from build123d import *

# Parameters (mm, degrees)
SKETCH1_R           = 2.4765
BOSS_EXTRUDE1_DEPTH = 1.524
SKETCH2_R           = 1.524
BOSS_EXTRUDE2_DEPTH = 18.161
CUT_EXTRUDE1_START  = -1.397
SKETCH4_R           = 1.524
CUT_EXTRUDE1_DEPTH  = 1.397
SKETCH5_R           = 1.4605
BOSS_EXTRUDE3_DEPTH = 0.381
SKETCH6_R           = 1.524
BOSS_EXTRUDE4_DEPTH = 1.016
FILLET1_R           = 0.635


with BuildPart() as part:
    # Sketch1 → Boss-Extrude1 (new body)
    with BuildSketch(Plane.XY):
        Circle(SKETCH1_R)
    extrude(amount=-BOSS_EXTRUDE1_DEPTH)

    # Sketch2 → Boss-Extrude2 (add)
    with BuildSketch(Plane(origin=(0, 0, -1.524), x_dir=(-1, 0, 0), z_dir=(0, 0, -1))):
        with Locations(Location((0, 0, 0), (0, 0, 180))):
            Circle(SKETCH2_R)
    extrude(amount=BOSS_EXTRUDE2_DEPTH)

    # Sketch4 → Cut-Extrude1 (cut)
    with BuildSketch(Plane(origin=(0, 0, -19.685), x_dir=(-1, 0, 0), z_dir=(0, 0, -1)).offset(CUT_EXTRUDE1_START)):
        with Locations(Location((0, 0, 0), (0, 0, 180))):
            Circle(SKETCH4_R)
    extrude(amount=CUT_EXTRUDE1_DEPTH, mode=Mode.SUBTRACT)

    # Sketch5 → Boss-Extrude3 (add)
    with BuildSketch(Plane(origin=(0, 0, -18.288), x_dir=(-1, 0, 0), z_dir=(0, 0, -1))):
        with Locations(Location((0, 0, 0), (0, 0, 180))):
            Circle(SKETCH5_R)
    extrude(amount=BOSS_EXTRUDE3_DEPTH)

    # Sketch6 → Boss-Extrude4 (add)
    with BuildSketch(Plane(origin=(0, 0, -18.669), x_dir=(-1, 0, 0), z_dir=(0, 0, -1))):
        with Locations(Location((0, 0, 0), (0, 0, 180))):
            Circle(SKETCH6_R)
    extrude(amount=BOSS_EXTRUDE4_DEPTH)

    # Fillet1
    fillet1_edges = [part.edges().sort_by_distance(p)[0] for p in [
        (-2.4765, 0, 0),
        (-2.4765, 0, -1.524),
    ]]
    fillet(fillet1_edges, radius=FILLET1_R)


solid = part.part
Check sheet for the modelled part. Datum: model origin and axes. Units: mm. A direction names the side the tool comes from. Give positions to 0.01 mm unless a question says otherwise; leave off trailing zeros. Write each loop counter-clockwise with the first axis right and the second up, starting at its lowest first coordinate (ties: lowest second). Pieces come first, ordered by that corner, then holes. Notation, with made-up numbers: (79, 35) -> (135, 35) arc R14 cw to (135, 45) -> close; hole circle Ø6 at (60.25, 4.25). An arc over 180 degrees is marked (long way). Write item = value, one per line.
Item 1: Sectioned sample at C-C on z = -10.5. Record the boundary of the cut face in (x, y).
Output:
outline = circle Ø3.05 at (0, 0)
Item 2: Release check for a two-part mould opening along Z. For faces 1 (the flat face through (0, 0, -19.685)), 2 (the cylindrical face through (-1.16, 0.89, -18.48)), 3 (the cylindrical face through (-0.2, -1.51, -9.79)) record: +Z half, -Z half, draft (parallel to the pull), parting line (faces both ways), or undercut.
Output:
face_1 = -Z half
face_2 = undercut
face_3 = draft
Item 3: Gauge pin test, flat end, axial feed: pin 1 (1.5 mm diameter, centred on y = 1, z = -8.5, fed in from -X). Record the tip position at first contact, or that the pin passes through.
Output:
pin_1 = -1.5
Item 4: Tool access check on faces 4 (the flat face through (0, 0, 0)), 5 (the cylindrical face through (-0.2, -1.51, -19.17)). Record the directions out of +Z, -Z, +X, -X, +Y, -Y that give a thin tool (end or side, any length) a straight path to the whole face; none if there is none.
Output:
face_4 = +Z, +X, -X, +Y, -Y
face_5 = -Z
Item 5: Scan lines: probe 1 along Y at (x, z) = (0.1, -5.75); probe 2 along Y at (x, z) = (0.7, -7.25); probe 3 along Z at (x, y) = (-1.9, 0.4). Record each from-to range of solid material in increasing order. Write a range as from..to.
Output:
probe_1 = -1.52..1.52
probe_2 = -1.35..1.35
probe_3 = -1.52..-0.01
